from build123d import *

# Parameters (mm, degrees)
SKETCH_1_W      = 3
SKETCH_1_H      = 38
SKETCH_1_W_2    = 104
EXTRUDE_1_DEPTH = 3
SKETCH_4_W      = 3
SKETCH_4_H      = 38
EXTRUDE_3_DEPTH = 107
FILLET_1_R      = 3
FILLET_2_R      = 3
FILLET_3_R      = 3
FILLET_5_R      = 3


with BuildPart() as part:
    # 草图1 → 凸台-拉伸1 (new body)
    with BuildSketch(Plane(origin=(0, 0, 0), x_dir=(1, 0, 0), z_dir=(0, 1, 0))):
        with Locations((-53.5, 0)):
            Rectangle(SKETCH_1_W, SKETCH_1_H)
        Rectangle(SKETCH_1_W_2, SKETCH_1_H)
        with Locations((53.5, 0)):
            Rectangle(SKETCH_1_W, SKETCH_1_H)
    extrude(amount=EXTRUDE_1_DEPTH)

    # 草图4 → 凸台-拉伸3 (add)
    with BuildSketch(Plane.XZ):
        with Locations((53.5, 0)):
            Rectangle(SKETCH_4_W, SKETCH_4_H)
        with Locations((-53.5, 0)):
            Rectangle(SKETCH_4_W, SKETCH_4_H)
    extrude(amount=EXTRUDE_3_DEPTH)

    # 圆角1
    fillet_1_edges = [part.edges().sort_by_distance(p)[0] for p in [
        (-55, 3, 0),
        (55, 3, 0),
    ]]
    fillet(fillet_1_edges, radius=FILLET_1_R)

    # 圆角2
    fillet_2_edges = [part.edges().sort_by_distance(p)[0] for p in [
        (52, 0, 0),
    ]]
    fillet(fillet_2_edges, radius=FILLET_2_R)

    # 圆角3
    fillet_3_edges = [part.edges().sort_by_distance(p)[0] for p in [
        (-52, 0, 0),
    ]]
    fillet(fillet_3_edges, radius=FILLET_3_R)

    # 圆角5
    fillet_5_edges = [part.edges().sort_by_distance(p)[0] for p in [
        (53.5, -107, -19),
        (-53.5, -107, -19),
    ]]
    fillet(fillet_5_edges, radius=FILLET_5_R)


solid = part.part
Verification items for the finished model (mm, model axes). A direction names the side the tool comes from. Give positions to 0.01 mm unless a question says otherwise; leave off trailing zeros. Loops run counter-clockwise (first coordinate to the right, second up) from the corner with the lowest first, then second, coordinate; pieces in that order, holes last. Notation, with made-up numbers: (44, 58.25) - (67, 58.25) arc R5 ccw to (67, 65.25) - close; hole circle Ø11 at (53, -33). An arc over 180 degrees is marked (long way). Write item = value, one per line. Start each with the question number.
Q1. Cross-section at B-B, the plane z = 0.5. Enter the section's corners in (x, y), and give its area (3 significant figures).
Q2. Thickness scan on line 1 (X direction, y = -51.5, z = -9.5); line 2 (Y direction, x = -21, z = -10). Record the ranges inside material, lowest first.
Q3. Cross-section at A-A, the plane y = -47. Enter the section's corners in (x, z), and give its area (3 significant figures).
Q4. Mould release check, pull along X, two halves, no side actions. Record for faces 1 (the face through (-55, -54, 0)), 2 (the face through (-54, -107, 2)), 3 (the face through (52, -54, 0)): released by +X, released by -X, zero draft, split by the parting line, or undercut.
Q5. Cross-section at C-C, the plane x = 41. Enter the section's corners in (y, z).
Q6. Tool access check on faces 4 (the face through (-53.48, -106.14, -18.1)), 5 (the face through (-1, 0, 0)). Record the directions out of +Z, -Z, +X, -X, +Y, -Y that give a thin tool (end or side, any length) a straight path to the whole face; none if there is none.
Answer key:
q1.outline = (-55, -107) - (-52, -107) - (-52, -3) arc R3 cw to (-49, 0) - (49, 0) arc R3 cw to (52, -3) - (52, -107) - (55, -107) - (55, 0) arc R3 ccw to (52, 3) - (-52, 3) arc R3 ccw to (-55, 0) - close
q1.area = 972 mm^2
q2.line_1 = -55 to -52, 52 to 55
q2.line_2 = 0 to 3
q3.outline = (-55, -19) - (-52, -19) - (-52, 19) - (-55, 19) - close; (52, -19) - (55, -19) - (55, 19) - (52, 19) - close
q3.area = 228 mm^2
q4.face_1 = released by -X
q4.face_2 = zero draft
q4.face_3 = undercut
q5.outline = (0, -19) - (3, -19) - (3, 19) - (0, 19) - close
q6.face_4 = -Z, +X, -X, -Y
q6.face_5 = +Z, -Z, -Y
